Build history of the part. All positions in model axes, mm. A direction names the side the tool comes from. Give positions to 0.01 mm unless a question says otherwise; leave off trailing zeros. Loops run counter-clockwise (first coordinate to the right, second up) from the corner with the lowest first, then second, coordinate; pieces in that order, holes last. Notation, with made-up numbers: M -25,-38.75 L 27,-38.75 A25 cw 27,-21.75 Z; hole C -22,-8 d5. An arc over 180 degrees is marked long. Answer as a JSON object with one key per item and string values. Group by question number.
1. 3-axis set-ups, long thin cutter, end or side, ignore diameter. For faces 3 (the face through (-13.399, 12.358, 26.156)), 4 (the face through (-15.436, 2.218, 20.785)): which of +Z, -Z, +X, -X, +Y, -Y reach the whole face in a straight line?
2. Slice it at A-A (z = 0). Give the number of separate pieces and of enclosed holes in the cut face, then the cut area to 4 significant figures.
3. Drop flat-ended pins along their axis: pin 1 Ø4.5 at (x, z) = (-14, 24.25) entering from -Y; pin 2 Ø5 at (x, y) = (24, 10.5) entering from +Z; pin 3 Ø2.5 at (x, z) = (0, -28) entering from -Y. Give the stop position or say it passes through.
4. Drill centre lines: line 1 along X through (y, z) = (2.55, 0); line 2 along Z through (x, y) = (13.5, 14.5); line 3 along X through (y, z) = (4, -14). Where is each one in solid material? Low to high. Write a range as [from, to].
5. Slice it at C-C (y = 16.5). List the corners of the cut face in (x, z), then the cut area to 3 significant figures.
6. Mould opens along X. For faces 1 (the face through (1.517, 3.451, -34.467)), 2 (the face through (-15.44, 2.22, -27.71)) say: released by +X, released by -X, zero draft, split by the parting line, or undercut.
7. Slice it at B-B (x = 0). List the corners of the cut face in (y, z).
from build123d import *

# Parameters (mm, degrees)
SKETCH_1_R          = 34.5
EXTRUDE_1_DEPTH     = 20
CUT_EXTRUDE_START   = -13
SKETCH_2_R          = 34.5
SKETCH_2_R_2        = 32.5
CUT_EXTRUDE_1_DEPTH = 13
SKETCH_3_R          = 2
CUT_EXTRUDE_3_DEPTH = 53.730446613
SKETCH_7_R          = 13
CUT_EXTRUDE_6_DEPTH = 53.730446613
SKETCH_8_R          = 3.75
CUT_EXTRUDE_7_DEPTH = 4.5
CHAMFER_4_SIZE      = 1
SKETCH_9_R          = 2
CUT_EXTRUDE_8_DEPTH = 10


with BuildPart() as part:
    # Sketch 1 → Extrude 1 (new body)
    with BuildSketch(Plane(origin=(0, 0, 0), x_dir=(1, 0, 0), z_dir=(0, 1, 0))):
        with Locations(Location((0, 0, 0), (0, 0, 270))):
            Circle(SKETCH_1_R)
    extrude(amount=EXTRUDE_1_DEPTH)

    # Sketch 2 → Cut-Extrude 1 (cut)
    with BuildSketch(Plane(origin=(0, 20, 0), x_dir=(1, 0, 0), z_dir=(0, 1, 0)).offset(CUT_EXTRUDE_START)):
        with Locations(Location((0, 0, 0), (0, 0, 270))):
            Circle(SKETCH_2_R)
        with Locations(Location((0, 0, 0), (0, 0, 270))):
            Circle(SKETCH_2_R_2, mode=Mode.SUBTRACT)
    extrude(amount=CUT_EXTRUDE_1_DEPTH, mode=Mode.SUBTRACT)

    # Sketch 3 → Cut-Extrude 3 (cut, through all)
    with BuildSketch(Plane(origin=(0, 20, 0), x_dir=(1, 0, 0), z_dir=(0, 1, 0))):
        with Locations(Location((-28, 0, 0), (0, 0, 270))):
            Circle(SKETCH_3_R)
        with Locations(Location((-14, 24.248711306, 0), (0, 0, 270))):
            Circle(SKETCH_3_R)
        with Locations(Location((14, 24.248711306, 0), (0, 0, 270))):
            Circle(SKETCH_3_R)
        with Locations(Location((28, 0, 0), (0, 0, 270))):
            Circle(SKETCH_3_R)
        with Locations(Location((14, -24.248711306, 0), (0, 0, 270))):
            Circle(SKETCH_3_R)
        with Locations(Location((-14, -24.248711306, 0), (0, 0, 270))):
            Circle(SKETCH_3_R)
    extrude(amount=-CUT_EXTRUDE_3_DEPTH, mode=Mode.SUBTRACT)

    # Sketch 7 → Cut-Extrude 6 (cut, through all)
    with BuildSketch(Plane(origin=(0, 20, 0), x_dir=(1, 0, 0), z_dir=(0, 1, 0))):
        with Locations(Location((0, 0, 0), (0, 0, 270))):
            Circle(SKETCH_7_R)
    extrude(amount=-CUT_EXTRUDE_6_DEPTH, mode=Mode.SUBTRACT)

    # Sketch 8 → Cut-Extrude 7 (cut)
    with BuildSketch(Plane.XZ):
        with Locations(Location((-28, 0, 0), (0, 0, 270))):
            Circle(SKETCH_8_R)
        with Locations(Location((-14, 24.248711306, 0), (0, 0, 270))):
            Circle(SKETCH_8_R)
        with Locations(Location((14, 24.248711306, 0), (0, 0, 270))):
            Circle(SKETCH_8_R)
        with Locations(Location((28, 0, 0), (0, 0, 270))):
            Circle(SKETCH_8_R)
        with Locations(Location((14, -24.248711306, 0), (0, 0, 270))):
            Circle(SKETCH_8_R)
        with Locations(Location((-14, -24.248711306, 0), (0, 0, 270))):
            Circle(SKETCH_8_R)
    extrude(amount=-CUT_EXTRUDE_7_DEPTH, mode=Mode.SUBTRACT)

    # Chamfer 4
    chamfer_4_edges = [part.edges().sort_by_distance(p)[0] for p in [
        (0, 20, -32.5),
    ]]
    chamfer(chamfer_4_edges, length=CHAMFER_4_SIZE)

    # Sketch 9 → Cut-Extrude 8 (cut)
    with BuildSketch(Plane.XZ):
        with Locations(Location((0, 28, 0), (0, 0, 270))):
            Circle(SKETCH_9_R)
        with Locations(Location((24.248711306, 14, 0), (0, 0, 270))):
            Circle(SKETCH_9_R)
        with Locations(Location((24.248711306, -14, 0), (0, 0, 270))):
            Circle(SKETCH_9_R)
        with Locations(Location((0, -28, 0), (0, 0, 270))):
            Circle(SKETCH_9_R)
        with Locations(Location((-24.248711306, -14, 0), (0, 0, 270))):
            Circle(SKETCH_9_R)
        with Locations(Location((-24.248711306, 14, 0), (0, 0, 270))):
            Circle(SKETCH_9_R)
    extrude(amount=-CUT_EXTRUDE_8_DEPTH, mode=Mode.SUBTRACT)


solid = part.part
Established:
{
 "1": {"face 3": "+Y, -Y", "face 4": "-Y"},
 "2": {"separate pieces": "4", "enclosed holes": "0", "area": "615.5 mm^2"},
 "3": {"pin 1": "stops at y = 4.5", "pin 2": "stops at z = 24.37", "pin 3": "stops at y = 10"},
 "4": {"line 1": "x = [-34.5, -31.75], [-24.25, -13], [13, 24.25], [31.75, 34.5]", "line 2": "z = [-29.56, -26.19], [-22.31, 22.31], [26.19, 29.56]", "line 3": "x = [-31.53, -26.25], [-22.25, 22.25], [26.25, 31.53]"},
 "5": {"outline": "C 0,0 d65; hole C -28,0 d4; hole C -14,-24.25 d4; hole C -14,24.25 d4; hole C 0,0 d26; hole C 14,-24.25 d4; hole C 14,24.25 d4; hole C 28,0 d4", "area": "2,710 mm^2"},
 "6": {"face 1": "split by the parting line", "face 2": "undercut"},
 "7": {"outline": "M 0,-34.5 L 7,-34.5 L 7,-32.5 L 19,-32.5 L 20,-31.5 L 20,-13 L 0,-13 L 0,-26 L 10,-26 L 10,-30 L 0,-30 Z; M 0,13 L 20,13 L 20,31.5 L 19,32.5 L 7,32.5 L 7,34.5 L 0,34.5 L 0,30 L 10,30 L 10,26 L 0,26 Z"}
}
